Autodesk Inventor part; units mm, degrees
ref_plane "YZ Plane" through (0, 0, 0) normal (1, 0, 0) x (0, 1, 0)
ref_plane "XZ Plane" through (0, 0, 0) normal (0, 1, 0) x (-1, 0, 0)
ref_plane "XY Plane" through (0, 0, 0) normal (0, 0, 1) x (1, 0, 0)
sketch "Sketch1" plane through (0, 0, 0) normal (0, 1, 0) x (-1, 0, 0)
  line L0 (140, 0) -> (74, 0)
  line L1 (74, 0) -> (76, 0)
  line L2 (140, 0) -> (140, -60)
  line L3 (140, -60) -> (140, 0)
  line L4 (138, -58) -> (82, -2)
  line L5 (82, -58) -> (138, -2)
  circle A0 centre (110, -30) radius 19.4
  circle A1 centre (104, -30) radius 19.4
  line L6 (110, -30) -> (110, -49.4)
  line L7 (86.45, -6.45) -> (86.45, -53.55)
  line L8 (82, -58) -> (82, -2)
  line L9 (76, -58) -> (76, -2)
  line L10 (74, 0) -> (74, -60)
  line L11 (74, 0) -> (74, -60)
  circle A2 centre (86.45, -6.45) radius 2.5
  line L12 (76, -2) -> (138, -2)
  line L13 (80.45, -8.95) -> (133.55, -8.95)
  line L14 (80.45, -3.95) -> (133.55, -3.95)
  line L15 (133.55, -6.45) -> (86.45, -6.45)
  line L16 (82, -2) -> (138, -2)
  line L17 (104, -10.6) -> (110, -10.6)
  line L18 (138, -2) -> (138, -58)
  line L19 (138, -2) -> (138, -58)
  line L20 (133.55, -53.55) -> (133.55, -6.45)
  line L21 (140, -60) -> (138, -60)
  line L22 (138, -60) -> (138, -58)
  line L23 (138, -58) -> (140, -58)
  line L24 (140, -58) -> (140, -60)
  line L25 (104, -49.4) -> (110, -49.4)
  circle A3 centre (86.45, -53.55) radius 2.5
  line L26 (133.55, -51.05) -> (80.45, -51.05)
  line L27 (86.45, -53.55) -> (133.55, -53.55)
  line L28 (80.45, -56.05) -> (133.55, -56.05)
  line L29 (138, -58) -> (82, -58)
  line L30 (138, -58) -> (76, -58)
  line L31 (74, -60) -> (140, -60)
  line L32 (140, -60) -> (32, -60)
  circle A4 centre (127.55, -53.55) radius 2.5
  line L33 (104, -30) -> (104, -49.4)
  circle A5 centre (80.45, -6.45) radius 2.5
  line L34 (86.45, -53.55) -> (82, -53.55)
  line L35 (82, -58) -> (86.45, -58)
  line L36 (86.45, -58) -> (86.45, -53.55)
  line L37 (82, -53.55) -> (82, -58)
  circle A6 centre (80.45, -53.55) radius 2.5
  circle A7 centre (133.55, -53.55) radius 2.5
  line L38 (76, 0) -> (76, -2)
  line L39 (76, -2) -> (74, -2)
  line L40 (74, -2) -> (74, 0)
  line L41 (138, -2) -> (133.55, -2)
  line L42 (133.55, -2) -> (133.55, -6.45)
  line L43 (133.55, -6.45) -> (138, -6.45)
  line L44 (138, -6.45) -> (138, -2)
  circle A8 centre (127.55, -6.45) radius 2.5
  circle A9 centre (133.55, -6.45) radius 2.5
  line L45 (0, -25) -> (0, 0)
  line L46 (32, -60) -> (0, -25)
  line L47 (0, -25) -> (0, 0)
  line L48 (0, 0) -> (74, 0)
  line L49 (0, 0) -> (74, 0)
  line L50 (140, -60) -> (140, 0)
  line L51 (140, -60) -> (0, -60)
  line L52 (0, -60) -> (0, 0)
  line L53 (0, 0) -> (140, 0)
  line L54 (140, 0) -> (140, -60)
  line L55 (0, -60) -> (40, -60)
  line L56 (40, -60) -> (40, -100)
  line L57 (40, -100) -> (0, -100)
  line L58 (0, -100) -> (0, -60)
  line L59 (138, -58) -> (128.5, -58)
  line L60 (128.5, -58) -> (128.5, -48.5)
  line L61 (128.5, -48.5) -> (138, -48.5)
  line L62 (138, -48.5) -> (138, -58)
  line L63 (82, -58) -> (91.5, -58)
  line L64 (91.5, -58) -> (91.5, -48.5)
  line L65 (91.5, -48.5) -> (82, -48.5)
  line L66 (82, -48.5) -> (82, -58)
  line L67 (138, -2) -> (128.5, -2)
  line L68 (128.5, -2) -> (128.5, -11.5)
  line L69 (128.5, -11.5) -> (138, -11.5)
  line L70 (138, -11.5) -> (138, -2)
  line L71 (82, -2) -> (91.5, -2)
  line L72 (91.5, -2) -> (91.5, -11.5)
  line L73 (91.5, -11.5) -> (82, -11.5)
  line L74 (82, -11.5) -> (82, -2)
  point P0 (127.55, 3.95)
  point P1 (127.55, 8.95)
  point P2 (86.45, 3.95)
  point P3 (86.45, 8.95)
  point P4 (127.55, 56.05)
  point P5 (127.55, 51.05)
  point P6 (86.45, 56.05)
  point P7 (86.45, 51.05)
  point P8 (123.7179, -16.2821)
  point P9 (131.05, -8.95)
  point P10 (88.95, -8.95)
  point P11 (88.2178, -8.2178)
  point P12 (86.45, -8.95)
  point P13 (82, -3.95)
  point P14 (135.3178, -55.3178)
  point P15 (127.55, -56.05)
  point P16 (127.55, -51.05)
  point P17 (131.05, -51.05)
  point P18 (123.7179, -43.7179)
  point P19 (86.45, -51.05)
  point P20 (86.45, -56.05)
  point P21 (86.45, -3.95)
  point P22 (127.55, -8.95)
  point P23 (127.55, -3.95)
  point P24 (86.45, -8.95)
  point P25 (86.45, -3.95)
  point P26 (127.55, -56.05)
  point P27 (127.55, -51.05)
  point P28 (127.55, -8.95)
  point P29 (127.55, -3.95)
  point P30 (86.45, -51.05)
  point P31 (86.45, -56.05)
  dimension "d0" = 40
  dimension "d1" = 40
  dimension "d2" = 9.5
  dimension "d3" = 9.5
  dimension "d4" = 9.5
  dimension "d5" = 9.5
  dimension "d6" = 9.5
  dimension "d7" = 9.5
  dimension "d8" = 9.5
  dimension "d9" = 9.5
extrude "Extrusion1" add sketch "Sketch1" along normal blind 10 contours L29 L60 L28 A7 L4 | L4 A7 L20 L61 L18 | L12 L72 L14 L4 | L4 L14 L8 | A7 L27 L4 | L4 L20 A7 | L61 L20 L69 L18 | L29 L64 L28 L60 | L8 L28 L5 | L5 L28 L36 L29 | L14 A2 L4 | L4 A2 L13 L8 A5 L14 | L12 L68 L14 L72 | L27 A7 L4 | L4 A7 L20 | L28 L60 A4 L27 A7 | L69 L20 A9 L43 L18 | L61 L4 A0 L5 L69 L20 | L20 L26 L4 L61 | L29 L36 L28 L64 | L28 A4 L60 | L28 L8 A6 L34 A3 L5 | L5 A3 L28 | A2 L15 L4 | L4 L7 A2 | L14 L72 L15 A2 | A5 L8 | L12 L42 L14 L68 | L14 A8 L15 L72 | A7 L27 A4 L60 L26 L4 | L4 L26 A7 | L43 A9 L5 L18 | L69 L5 L13 L20 | L60 L26 L64 L5 A1 L25 A0 L4 | L4 L26 L60 | L64 L27 A4 L28 | L28 A3 L27 L64 | A4 L27 L60 | L60 L27 A4 | A3 L34 L5 | L5 L36 A3 | L36 L27 A3 | L8 L34 A6 | L15 A2 L4 | L4 A2 L7 | L13 L4 L73 L7 | L7 L73 L8 L13 | A2 L4 L13 | L15 L72 L13 L4 A2 | L12 L5 A9 L42 | L68 A8 L14 | L14 A9 L15 A8 L68 | A8 L68 L15 | L15 A8 L13 L72 | L27 L60 A4 | A9 L20 L43 | L43 L5 A9 | A9 L5 L20 | L13 L5 A9 | L68 L13 L5 | L5 A0 L17 A1 L4 L72 L13 L68 | A0 L6 A1 L4 | L4 A1 L5 A0 | L60 A4 L26 | L64 L26 A4 L27 | L27 A3 L5 L26 L64 | A4 L60 L27 | L7 A3 L5 | L34 A3 L7 | L5 A3 L27 | L34 A6 L8 L26 A3 | L8 A6 L34 | L73 L4 A1 L7 | L7 A1 L65 L8 L73 | L13 L72 L4 | A9 L5 L42 | L42 L15 A9 | A8 L15 L68 | L15 L68 A8 | L5 A9 L15 | L13 L68 A8 L15 A9 L5 | L5 A1 A0 | L13 A8 L68 | A1 L6 L4 | L4 L5 A1 | L25 A1 A0 | A0 A1 L6 | L26 L5 L64 | A3 L26 L5 | L26 L8 L65 L7 | L7 L65 L5 L26 | L7 A1 | A1 L4 A0 L5 L7 | A8 L68 L15 | L5 L4 A0 A1 | A0 A1 L17 | L5 A0 L4 | L6 A1 A0 L33 L5 | A1 L33 A0 | A1 L5 A0 L33 | L65 L7 A1 L5 | A1 A0 L4 | L33 A0 L5 picked at (82.1331, -6.9717)
sketch "Sketch2" plane through (0, 10, 0) normal (0, 1, 0) x (1, 0, 0)
  line L0 (-82, 58) -> (-138, 58)
  line L1 (-138, 2) -> (-82, 2)
  line L2 (-138, 58) -> (-82, 58)
  line L3 (-82, 58) -> (-82, 2)
  line L4 (-82, 2) -> (-138, 2)
  line L5 (-138, 2) -> (-138, 58)
  line L6 (-138, 58) -> (-138, 2)
  line L7 (-138, 58) -> (-129, 58)
  line L8 (-129, 58) -> (-129, 49)
  line L9 (-129, 49) -> (-138, 49)
  line L10 (-138, 49) -> (-138, 58)
  line L11 (-82, 58) -> (-91, 58)
  line L12 (-91, 58) -> (-91, 49)
  line L13 (-91, 49) -> (-82, 49)
  line L14 (-82, 49) -> (-82, 58)
  line L15 (-138, 2) -> (-129, 2)
  line L16 (-129, 2) -> (-129, 11)
  line L17 (-129, 11) -> (-138, 11)
  line L18 (-138, 11) -> (-138, 2)
  line L19 (-82, 2) -> (-91, 2)
  line L20 (-91, 2) -> (-91, 11)
  line L21 (-91, 11) -> (-82, 11)
  line L22 (-82, 11) -> (-82, 2)
  line L23 (-140, 0) -> (-74, 0)
  line L24 (-74, 0) -> (-76, 0)
  line L25 (-140, 0) -> (-140, 60)
  line L26 (-140, 60) -> (-140, 0)
  line L27 (-138, 58) -> (-82, 2)
  line L28 (-82, 58) -> (-138, 2)
  circle A0 centre (-110, 30) radius 19.4
  circle A1 centre (-104, 30) radius 19.4
  line L29 (-110, 30) -> (-110, 49.4)
  line L30 (-86.45, 6.45) -> (-86.45, 53.55)
  line L31 (-82, 58) -> (-82, 2)
  line L32 (-76, 58) -> (-76, 2)
  line L33 (-74, 0) -> (-74, 60)
  line L34 (-74, 0) -> (-74, 60)
  circle A2 centre (-86.45, 6.45) radius 2.5
  line L35 (-76, 2) -> (-138, 2)
  line L36 (-80.45, 8.95) -> (-133.55, 8.95)
  line L37 (-80.45, 3.95) -> (-133.55, 3.95)
  line L38 (-133.55, 6.45) -> (-86.45, 6.45)
  line L39 (-82, 2) -> (-138, 2)
  line L40 (-104, 10.6) -> (-110, 10.6)
  line L41 (-138, 2) -> (-138, 58)
  line L42 (-138, 2) -> (-138, 58)
  line L43 (-133.55, 53.55) -> (-133.55, 6.45)
  line L44 (-140, 60) -> (-138, 60)
  line L45 (-138, 60) -> (-138, 58)
  line L46 (-138, 58) -> (-140, 58)
  line L47 (-140, 58) -> (-140, 60)
  line L48 (-104, 49.4) -> (-110, 49.4)
  circle A3 centre (-86.45, 53.55) radius 2.5
  line L49 (-133.55, 51.05) -> (-80.45, 51.05)
  line L50 (-86.45, 53.55) -> (-133.55, 53.55)
  line L51 (-80.45, 56.05) -> (-133.55, 56.05)
  line L52 (-138, 58) -> (-82, 58)
  line L53 (-138, 58) -> (-76, 58)
  line L54 (-74, 60) -> (-140, 60)
  line L55 (-140, 60) -> (-32, 60)
  circle A4 centre (-127.55, 53.55) radius 2.5
  line L56 (-104, 30) -> (-104, 49.4)
  circle A5 centre (-80.45, 6.45) radius 2.5
  line L57 (-86.45, 53.55) -> (-82, 53.55)
  line L58 (-82, 58) -> (-86.45, 58)
  line L59 (-86.45, 58) -> (-86.45, 53.55)
  line L60 (-82, 53.55) -> (-82, 58)
  circle A6 centre (-80.45, 53.55) radius 2.5
  circle A7 centre (-133.55, 53.55) radius 2.5
  line L61 (-76, 0) -> (-76, 2)
  line L62 (-76, 2) -> (-74, 2)
  line L63 (-74, 2) -> (-74, 0)
  line L64 (-138, 2) -> (-133.55, 2)
  line L65 (-133.55, 2) -> (-133.55, 6.45)
  line L66 (-133.55, 6.45) -> (-138, 6.45)
  line L67 (-138, 6.45) -> (-138, 2)
  circle A8 centre (-127.55, 6.45) radius 2.5
  circle A9 centre (-133.55, 6.45) radius 2.5
  line L68 (0, 25) -> (0, 0)
  line L69 (-32, 60) -> (0, 25)
  line L70 (0, 25) -> (0, 0)
  line L71 (0, 0) -> (-74, 0)
  line L72 (0, 0) -> (-74, 0)
  line L73 (-140, 60) -> (-140, 0)
  line L74 (-140, 60) -> (0, 60)
  line L75 (0, 60) -> (0, 0)
  line L76 (0, 0) -> (-140, 0)
  line L77 (-140, 0) -> (-140, 60)
  line L78 (0, 60) -> (-40, 60)
  line L79 (-40, 60) -> (-40, 100)
  line L80 (-40, 100) -> (0, 100)
  line L81 (0, 100) -> (0, 60)
  line L82 (-138, 58) -> (-128.5, 58)
  line L83 (-128.5, 58) -> (-128.5, 48.5)
  line L84 (-128.5, 48.5) -> (-138, 48.5)
  line L85 (-138, 48.5) -> (-138, 58)
  line L86 (-82, 58) -> (-91.5, 58)
  line L87 (-91.5, 58) -> (-91.5, 48.5)
  line L88 (-91.5, 48.5) -> (-82, 48.5)
  line L89 (-82, 48.5) -> (-82, 58)
  line L90 (-138, 2) -> (-128.5, 2)
  line L91 (-128.5, 2) -> (-128.5, 11.5)
  line L92 (-128.5, 11.5) -> (-138, 11.5)
  line L93 (-138, 11.5) -> (-138, 2)
  line L94 (-82, 2) -> (-91.5, 2)
  line L95 (-91.5, 2) -> (-91.5, 11.5)
  line L96 (-91.5, 11.5) -> (-82, 11.5)
  line L97 (-82, 11.5) -> (-82, 2)
  point P0 (127.55, 3.95)
  point P1 (127.55, 8.95)
  point P2 (86.45, 3.95)
  point P3 (86.45, 8.95)
  point P4 (127.55, 56.05)
  point P5 (127.55, 51.05)
  point P6 (86.45, 56.05)
  point P7 (86.45, 51.05)
  point P8 (123.7179, -16.2821)
  point P9 (131.05, -8.95)
  point P10 (88.95, -8.95)
  point P11 (88.2178, -8.2178)
  point P12 (86.45, -8.95)
  point P13 (82, -3.95)
  point P14 (82, -2)
  point P15 (74, -2)
  point P16 (138, -60)
  point P17 (135.3178, -55.3178)
  point P18 (127.55, -56.05)
  point P19 (127.55, -51.05)
  point P20 (131.05, -51.05)
  point P21 (123.7179, -43.7179)
  point P22 (86.45, -51.05)
  point P23 (86.45, -56.05)
  point P24 (86.45, -3.95)
  point P25 (127.55, -8.95)
  point P26 (127.55, -3.95)
  point P27 (0, -25)
  point P28 (40, -60)
  point P29 (86.45, -8.95)
  point P30 (86.45, -3.95)
  point P31 (127.55, -56.05)
  point P32 (127.55, -51.05)
  point P33 (127.55, -8.95)
  point P34 (127.55, -3.95)
  point P35 (0, -25)
  point P36 (40, -60)
  point P37 (138, -60)
  point P38 (86.45, -51.05)
  point P39 (86.45, -56.05)
  point P40 (82, -2)
  point P41 (-91, 2)
  point P42 (-82, 11)
  point P43 (-138, 11)
  point P44 (-129, 2)
  dimension "d12" = 9
  dimension "d13" = 9
  dimension "d14" = 9
  dimension "d15" = 9
  dimension "d16" = 9
  dimension "d17" = 9
  dimension "d18" = 9
  dimension "d19" = 9
  dimension "d20" = 40
  dimension "d21" = 40
  dimension "d22" = 9.5
  dimension "d23" = 9.5
  dimension "d24" = 9.5
  dimension "d25" = 9.5
  dimension "d26" = 9.5
  dimension "d27" = 9.5
  dimension "d28" = 9.5
  dimension "d29" = 9.5
extrude "Extrusion2" add sketch "Sketch2" along normal blind 10 contours L28 L51 L59 L0 | L3 L51 L28 | L59 L51 L12 L0 | L3 A6 L57 A3 L28 L51 | L28 A3 L51 | A3 L50 L12 L51 | L3 L57 A6 | A3 L28 L49 L12 L50 | L3 A6 L57 | A6 L3 L49 A3 L57 | L27 L37 L3 | L1 L20 L37 L27 | A3 L49 L28 | L49 L3 L13 L30 | L30 L13 L28 L49 | L37 L27 A2 L36 L3 A5 | L37 A2 L27 | L8 L51 A7 L27 L0 | L49 L28 L12 | L20 L38 A2 L37 | A5 L3 | L27 A7 L43 L9 L5 | L8 A4 L50 A7 L51 | L20 L36 L27 A2 L38 | L8 L50 A4 | L1 L65 L37 L16 | L20 L27 L36 | L36 L30 L21 L3 | L27 L36 A2 | L36 L27 L21 L30 | L43 L49 L27 L9 | A7 L27 L49 | L8 A4 L50 | A4 L8 L49 L27 A7 L50 | L1 L28 A9 L65 | L37 A9 L38 A8 L16 | L27 L49 L8 | L5 L66 A9 L28 | A8 L38 L16 | L17 L43 A9 L66 L5 | A9 L28 L36 L16 A8 L38 | L38 A8 L16 | L17 L28 L36 L43 | A9 L36 L28 | L36 L28 L16 picked at (-82.2333, 6.0868)
fillet "Fillet1" radius 5.5 4 edges at (-91, 15, -49) (-129, 15, -49) (-129, 15, -11) (-91, 15, -11)
fillet "Fillet2" radius 2 12 edges at (-82, 10, -2) (-138, 10, -2) (-138, 10, -58) (-82, 10, -58) (-91, 15, -58) (-82, 15, -49) (-129, 15, -58) (-138, 15, -49) (-138, 15, -11) (-129, 15, -2) (-91, 15, -2) (-82, 15, -11)
sketch "Sketch3" plane through (0, 20, 0) normal (0, 1, 0) x (1, 0, 0)
  circle A0 centre (-133.55, 53.55) radius 2.5
  circle A1 centre (-133.55, 53.55) radius 2.5
  circle A2 centre (-86.45, 53.55) radius 2.5
  circle A3 centre (-86.45, 53.55) radius 2.5
  circle A4 centre (-133.55, 6.45) radius 2.5
  circle A5 centre (-133.55, 6.45) radius 2.5
  circle A6 centre (-86.45, 6.45) radius 2.5
  circle A7 centre (-86.45, 6.45) radius 2.5
  point P0 (0, 0)
extrude "Extrusion3" cut sketch "Sketch3" against normal through all
properties part number "duzy_silnik_tyl"
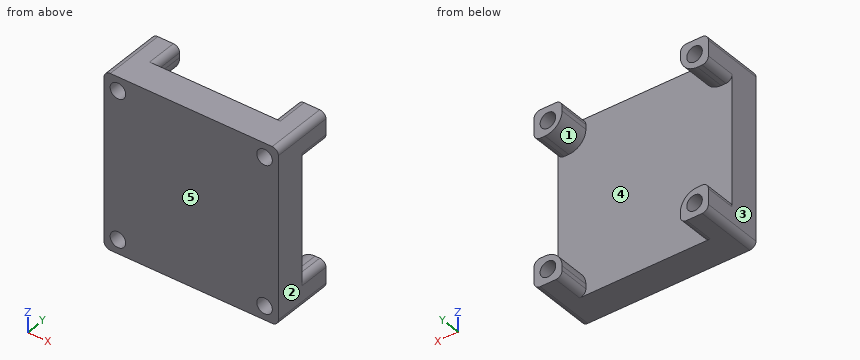
Geometry check sheet. Reference: the model listing, model coordinates, mm. Face numbers are marked on the shaded views. A direction names the side the tool comes from. Coordinates: 2 decimals unless noted, no trailing zeros. Loops run counter-clockwise (first coordinate to the right, second up) from the corner with the lowest first, then second, coordinate; pieces in that order, holes last. Notation, with made-up numbers: (14, 36) - (23, 36) arc R34 cw to (23, 71) - close; hole circle Ø5 at (44.25, -25.75). An arc over 180 degrees is marked (long way). One line per item, written item: value. Start each with the question number.
(1) Cross-section at C-C on z = -53.55. Enter the section's corners in (x, y).
(2) Material ranges on line 1 (Z direction, x = -133.55, y = 4.5); line 2 (X direction, y = 8.75, z = -6.45); line 3 (Y direction, x = -91, z = -26.5), recorded low to high. Write a range as [from, to].
(3) Tool access check on the marked faces 4 and 5. Record the directions out of +Z, -Z, +X, -X, +Y, -Y that give a thin tool (end or side, any length) a straight path to the whole face; none if there is none.
(4) Mould release check, pull along X, two halves, no side actions. Record for the marked faces 1, 2 and 3: released by +X, released by -X, zero draft, split by the parting line, or undercut.
(5) Cross-section at B-B on x = -133.55. Enter the section's corners in (y, z).
(6) Cross-section at D-D on y = 17. Count the separate pieces of the cut face and the enclosed holes in it, plus the area to 3 significant figures.
(7) Cross-section at A-A on y = 4.75. Enter the section's corners in (x, z).
(8) Depth check by flat-ended pin: P1, Ø1.5, axis at x = -109.5, z = -20.5, coming from the -Y side; P2, Ø10, axis at y = 16.5, z = -40.5, coming from the +X side. Enter the tip coordinate at first touch or a pass-through.
Results below:
1. outline: (-138, 0) - (-136.05, 0) - (-136.05, 20) - (-138, 20) - close; (-131.05, 0) - (-88.95, 0) - (-88.95, 20) - (-90.92, 20) - (-90.92, 10) - (-129.08, 10) - (-129.08, 20) - (-131.05, 20) - close; (-83.95, 0) - (-82, 0) - (-82, 20) - (-83.95, 20) - close
2. line 1: z = [-58, -56.05], [-51.05, -8.95], [-3.95, -2]
2. line 2: x = [-138, -136.05], [-131.05, -88.95], [-83.95, -82]
2. line 3: y = [0, 10]
3. face 4: +Y
3. face 5: +Z, -Z, +X, -X, -Y
4. face 1: undercut
4. face 2: released by +X
4. face 3: released by -X
5. outline: (0, -58) - (20, -58) - (20, -56.05) - (0, -56.05) - close; (0, -51.05) - (20, -51.05) - (20, -49.08) - (10, -49.08) - (10, -10.92) - (20, -10.92) - (20, -8.95) - (0, -8.95) - close; (0, -3.95) - (20, -3.95) - (20, -2) - (0, -2) - close
6. separate pieces: 4
6. enclosed holes: 4
6. area: 209 mm2
7. outline: (-138, -56) arc R2 ccw to (-136, -58) - (-84, -58) arc R2 ccw to (-82, -56) - (-82, -4) arc R2 ccw to (-84, -2) - (-136, -2) arc R2 ccw to (-138, -4) - close; hole circle Ø5 at (-133.55, -53.55); hole circle Ø5 at (-133.55, -6.45); hole circle Ø5 at (-86.45, -53.55); hole circle Ø5 at (-86.45, -6.45)
8. P1: stops at y = 0
8. P2: passes through
